Part print with two shaded views. Sizes in mm from the minimum x, y, z corner. A direction names the side the tool comes from. Round coordinates to 2 decimals unless told otherwise and drop trailing zeros. Order: outer loops, then holes, each group sorted by start corner. A loop starts at its lowest first (then second) coordinate and runs counter-clockwise, first axis right, second up. Notation, with made-up numbers: M -1,67 L 23,67 A13 ccw 23,85 Z; hole C 60.25,-20 d1. An arc over 180 degrees is marked long. One line per question, with ' | ' between items.
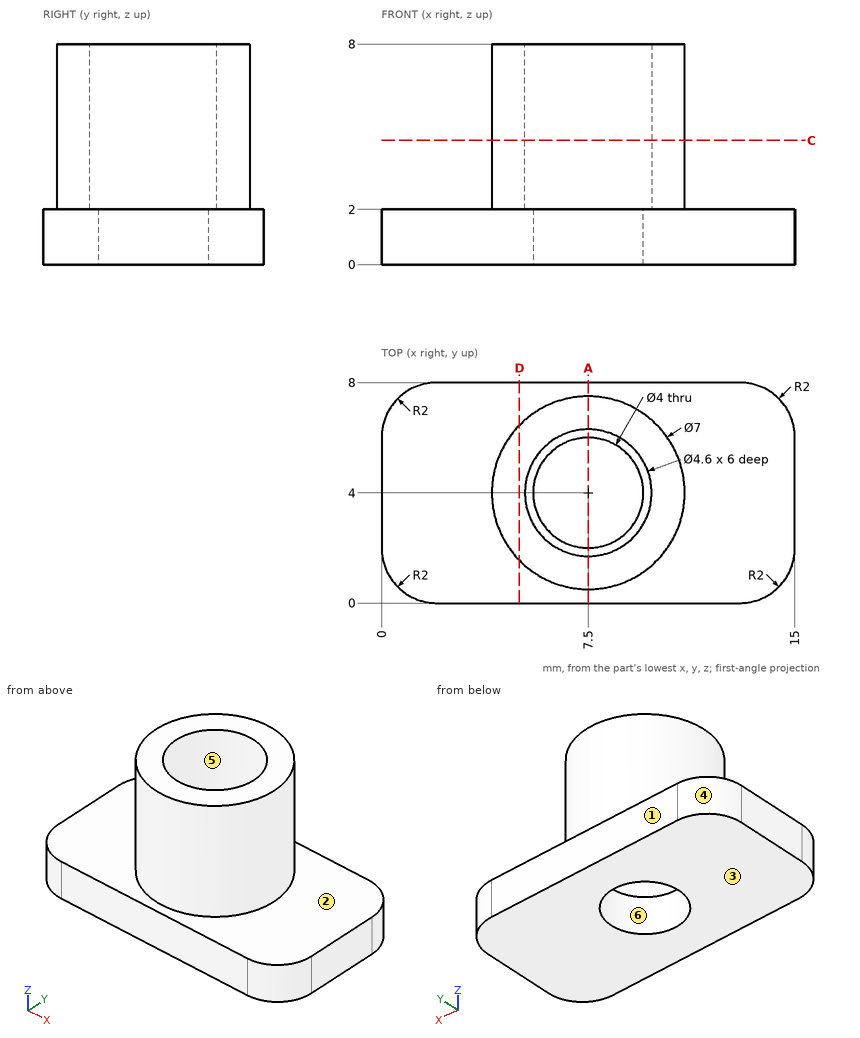
1) Saw through at C-C (z = 4.5). List the corners of the cut face in (x, y), plus the area to 3 significant figures.
The answers:
outline: C 7.5,4 d7; hole C 7.5,4 d4.6 | area: 21.9 mm²
2) Drop flat-ended pins along their axis: pin 1 (4 mm diameter, centred on x = 5.5, y = 3.5, fed in from +Z); pin 2 (3 mm diameter, centred on y = 6.5, z = 5.5, fed in from -X); pin 3 (1 mm diameter, centred on x = 12, z = 5, fed in from -Y); pin 4 (1.5 mm diameter, centred on y = 2, z = 7, fed in from +X). Give the stop position or say it passes through.
The answers:
pin 1: stops at z = 8 | pin 2: stops at x = 4.15 | pin 3: passes through | pin 4: stops at x = 10.77
3) Probe line 1 (Y direction, x = 7.5, z = 1.55); line 2 (Y direction, x = 7.5, z = 5.95); line 3 (Z direction, x = 4, y = 6.5). List the from-to ranges inside material, lowest first. Write a range as [from, to].
The answers:
line 1: y = [0, 2], [6, 8] | line 2: y = [0.5, 1.7], [6.3, 7.5] | line 3: z = [0, 2]
4) Two-plate mould, pull along Y, no slides. Class the marked faces 3, 4, 5 and 6: released by +Y, released by -Y, zero draft, split by the parting line, or undercut.
The answers:
face 3: zero draft | face 4: released by +Y | face 5: undercut | face 6: undercut
5) Which spindle directions (+Z, -Z, +X, -X, +Y, -Y) get a long thin tool onto all of the face, cutting with end or side? Do the marked faces 1 and 2. Say none if no direction does.
The answers:
face 1: +Z, -Z, +X, -X, +Y | face 2: +Z
6) Saw through at A-A (x = 7.5). List the corners of the cut face in (y, z).
The answers:
outline: M 0,0 L 2,0 L 2,2 L 1.7,2 L 1.7,8 L 0.5,8 L 0.5,2 L 0,2 Z; M 6,0 L 8,0 L 8,2 L 7.5,2 L 7.5,8 L 6.3,8 L 6.3,2 L 6,2 Z
7) Saw through at D-D (x = 5). List the corners of the cut face in (y, z), plus the area to 3 significant figures.
The answers:
outline: M 0,0 L 8,0 L 8,2 L 6.45,2 L 6.45,8 L 1.55,8 L 1.55,2 L 0,2 Z | area: 45.4 mm²
